```python
from build123d import *

# Parameters (mm, degrees)
F0_W     = 75
F0_H     = 134
F0_R     = 11.25
F1_DEPTH = 1.5


with BuildPart() as f1:
    # F0 (on Front) → F1 (new body)
    with BuildSketch(Plane.XZ):
        Rectangle(F0_W, F0_H)
        with Locations((0, -45)):
            Circle(F0_R, mode=Mode.SUBTRACT)
        with Locations((0, -15)):
            Circle(F0_R, mode=Mode.SUBTRACT)
        with Locations((0, 15)):
            Circle(F0_R, mode=Mode.SUBTRACT)
        with Locations((0, 45)):
            Circle(F0_R, mode=Mode.SUBTRACT)
    extrude(amount=F1_DEPTH)


solid = f1.part
```
Here's how the part is built. I have some questions about the finished solid (model axes, mm). Give positions to 0.01 mm unless a question says otherwise; leave off trailing zeros. Write each loop counter-clockwise with the first axis right and the second up, starting at its lowest first coordinate (ties: lowest second). Pieces come first, ordered by that corner, then holes.
(1) Imagine slicing it at A-A, the plane z = -45. Write out the boundary of the cut face in (x, y), and give its area (4 significant figures).
Output values:
outline: (-37.5, -1.5) - (-11.25, -1.5) - (-11.25, 0) - (-37.5, 0) - close; (11.25, -1.5) - (37.5, -1.5) - (37.5, 0) - (11.25, 0) - close
area: 78.75 mm2
(2) If I drill on L1, parallel to Z at x = 0, y = -1.2; L2, parallel to X at y = -0.2, z = -15.5; L3, parallel to Z at x = -10, y = -1.3, over which ranges is the centre line in solid material (lowest first)?
Output values:
L1: z = -67 to -56.25, -33.75 to -26.25, -3.75 to 3.75, 26.25 to 33.75, 56.25 to 67
L2: x = -37.5 to -11.24, 11.24 to 37.5
L3: z = -67 to -50.15, -39.85 to -20.15, -9.85 to 9.85, 20.15 to 39.85, 50.15 to 67
(3) Imagine slicing it at D-D, the plane x = 10. Write out the boundary of the cut face in (y, z).
Output values:
outline: (-1.5, -67) - (0, -67) - (0, -50.15) - (-1.5, -50.15) - close; (-1.5, -39.85) - (0, -39.85) - (0, -20.15) - (-1.5, -20.15) - close; (-1.5, -9.85) - (0, -9.85) - (0, 9.85) - (-1.5, 9.85) - close; (-1.5, 20.15) - (0, 20.15) - (0, 39.85) - (-1.5, 39.85) - close; (-1.5, 50.15) - (0, 50.15) - (0, 67) - (-1.5, 67) - close
(4) Imagine slicing it at C-C, the plane x = 0. Write out the boundary of the cut face in (y, z), and give its area (3 significant figures).
Output values:
outline: (-1.5, -67) - (0, -67) - (0, -56.25) - (-1.5, -56.25) - close; (-1.5, -33.75) - (0, -33.75) - (0, -26.25) - (-1.5, -26.25) - close; (-1.5, -3.75) - (0, -3.75) - (0, 3.75) - (-1.5, 3.75) - close; (-1.5, 26.25) - (0, 26.25) - (0, 33.75) - (-1.5, 33.75) - close; (-1.5, 56.25) - (0, 56.25) - (0, 67) - (-1.5, 67) - close
area: 66.0 mm2
(5) Thinking about a two-plate mould opening in Z: for faces 1 (the face through (-1, -1.5, 1)), 2 (the face through (-1.465, -0.74, -33.846)), which applies, pulls with the +Z half, pulls with the -Z half, needs draft (parallel to the pull), parting line crosses it, or undercut?
Output values:
face 1: needs draft
face 2: undercut
(6) Will this pin go through, and if not, where does the flat tip stop? pin 1 (6 mm diameter, centred on x = -18, z = 5.5, fed in from +Y).
Output values:
pin 1: stops at y = 0
(7) Imagine slicing it at B-B, the plane y = -0.3. Write out the boundary of the cut face in (x, z).
Output values:
outline: (-37.5, -67) - (37.5, -67) - (37.5, 67) - (-37.5, 67) - close; hole circle Ø22.5 at (0, -45); hole circle Ø22.5 at (0, -15); hole circle Ø22.5 at (0, 15); hole circle Ø22.5 at (0, 45)
